```python
from build123d import *

# Parameters (mm, degrees)
F0_R     = 2.5
F0_W     = 20
F0_H     = 3
F1_DEPTH = 10
F2_SIZE  = 2
F3_DEPTH = 8.5


with BuildPart() as f1:
    # F0 (on Top) → F1 (new body)
    with BuildSketch(Plane.XY):
        with BuildLine():
            ThreePointArc((-45, -10), (-42.0710678119, -17.0710678119), (-35, -20))
            Line((-35, -20), (35, -20))
            ThreePointArc((35, -20), (42.0710678119, -17.0710678119), (45, -10))
            Line((45, -10), (45, 102.6))
            ThreePointArc((45, 102.6), (42.0710678119, 109.6710678119), (35, 112.6))
            Line((35, 112.6), (-35, 112.6))
            ThreePointArc((-35, 112.6), (-42.0710678119, 109.6710678119), (-45, 102.6))
            Line((-45, 102.6), (-45, -10))
        make_face()
        with Locations((-35, -10)):
            Circle(F0_R, mode=Mode.SUBTRACT)
        with Locations((35, -10)):
            Circle(F0_R, mode=Mode.SUBTRACT)
        with Locations((-35, 102.6)):
            Circle(F0_R, mode=Mode.SUBTRACT)
        with BuildLine():
            ThreePointArc((-30, 74.7005903715), (-23.489485432, 87.4662673094), (-10.1106179057, 92.6))
            Line((-10.1106179057, 92.6), (-10, 92.6))
            Line((-10, 92.6), (-10, 95.6))
            Line((-10, 95.6), (10, 95.6))
            Line((10, 95.6), (10, 92.6))
            Line((10, 92.6), (10.1106179057, 92.6))
            ThreePointArc((10.1106179057, 92.6), (23.489485432, 87.4662673094), (30, 74.7005903715))
            Line((30, 74.7005903715), (36.9557528377, 8.8402361486))
            ThreePointArc((36.9557528377, 8.8402361486), (34.9465069238, 2.6484529895), (29, 0))
            Line((29, 0), (-29, 0))
            ThreePointArc((-29, 0), (-34.9465069238, 2.6484529895), (-36.9557528377, 8.8402361486))
            Line((-36.9557528377, 8.8402361486), (-30, 74.7005903715))
        make_face(mode=Mode.SUBTRACT)
        with Locations((35, 102.6)):
            Circle(F0_R, mode=Mode.SUBTRACT)
        with Locations((0, 94.1)):
            Rectangle(F0_W, F0_H)
    extrude(amount=F1_DEPTH)

    # F2
    f2_edges = [f1.edges().sort_by_distance(p)[0] for p in [
        (-37.5, -10, 10),
        (32.5, -10, 10),
        (32.5, 102.6, 10),
        (-37.5, 102.6, 10),
    ]]
    chamfer(f2_edges, length=F2_SIZE)

    # F0 (on Top) → F3 (cut)
    with BuildSketch(Plane.XY):
        with Locations((0, 94.1)):
            Rectangle(F0_W, F0_H)
    extrude(amount=F3_DEPTH, mode=Mode.SUBTRACT)


solid = f1.part
```
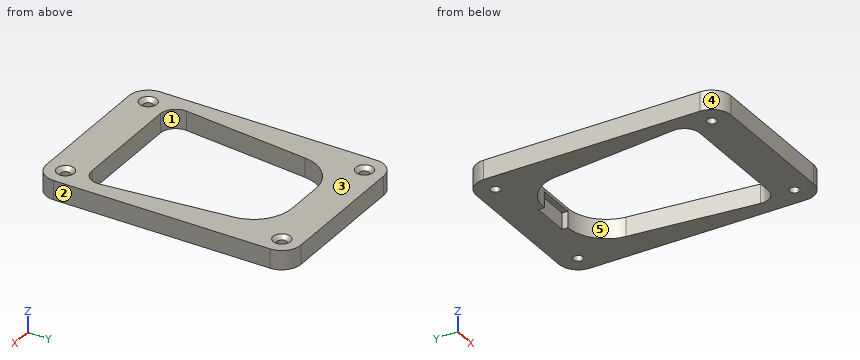
Geometry: final body of the model. Coordinates: model frame, mm. Face numbers are marked on the shaded views. A direction names the side the tool comes from. Round coordinates to 2 decimals unless told otherwise and drop trailing zeros. Order: outer loops, then holes, each group sorted by start corner. A loop starts at its lowest first (then second) coordinate and runs counter-clockwise, first axis right, second up. Notation, with made-up numbers: (74, 69.5) -> (101, 69.5) arc R20 ccw to (101, 103.5) -> close; hole circle Ø8 at (79, 65.5). An arc over 180 degrees is marked (long way). Write each question's results on one line, items separated by ' | '.
Q1. Pull-direction query (Y, two-part tool) for the marked faces 3, 4 and 5; classes: released by +Y, released by -Y, zero draft, split by the parting line, or undercut.
Response values:
face 3: zero draft | face 4: released by -Y | face 5: undercut
Q2. Section query C-C (y = 91). Output: boundary loops of the cut face in (x, z), and give its area (3 significant figures).
Response values:
outline: (-45, 0) -> (-17.95, 0) -> (-17.95, 10) -> (-45, 10) -> close; (17.95, 0) -> (45, 0) -> (45, 10) -> (17.95, 10) -> close | area: 541 mm²
Q3. Section query B-B (x = -24.5). Output: boundary loops of the cut face in (y, z), and give its area (3 significant figures).
Response values:
outline: (-20, 0) -> (0, 0) -> (0, 10) -> (-20, 10) -> close; (86.49, 0) -> (112.6, 0) -> (112.6, 10) -> (86.49, 10) -> close | area: 461 mm²
Q4. Pin query (flat end, axial travel): pin 1 Ø6.5 at (x, y) = (-35, 102.6) entering from +Z. Return the tip coordinate at first contact, or that it passes through.
Response values:
pin 1: z = 8.75
Q5. Ray query, line 1 along Y through (x, z) = (-5, 3); line 2 along Y through (x, z) = (-11, 1.5); line 3 along X through (y, z) = (37, 3). Return the intervals inside material, ascending.
Response values:
line 1: -20 to 0, 95.6 to 112.6 | line 2: -20 to 0, 92.58 to 112.6 | line 3: -45 to -33.98, 33.98 to 45
Q6. Access query for the marked faces 1 and 2. Directions: +Z, -Z, +X, -X, +Y, -Y. A direction counts if a zero-diameter tool reaches every point of the face in a straight line with its end or side. Return the directions, or none.
Response values:
face 1: +Z, -Z | face 2: +Z, -Z, +X, +Y, -Y
Q7. Section query A-A (z = 3.25). Output: boundary loops of the cut face in (x, y), and give its area (3 significant figures).
Response values:
outline: (-45, -10) arc R10 ccw to (-35, -20) -> (35, -20) arc R10 ccw to (45, -10) -> (45, 102.6) arc R10 ccw to (35, 112.6) -> (-35, 112.6) arc R10 ccw to (-45, 102.6) -> close; hole circle Ø5 at (-35, -10); hole circle Ø5 at (-35, 102.6); hole (-36.96, 8.84) arc R8 ccw to (-29, 0) -> (29, 0) arc R8 ccw to (36.96, 8.84) -> (30, 74.7) arc R20 ccw to (10.11, 92.6) -> (10, 92.6) -> (10, 95.6) -> (-10, 95.6) -> (-10, 92.6) -> (-10.11, 92.6) arc R20 ccw to (-30, 74.7) -> close; hole circle Ø5 at (35, -10); hole circle Ø5 at (35, 102.6) | area: 5,770 mm²
